Check sheet for the drawn part. Datum: minimum x, y, z corner. Units: mm. A direction names the side the tool comes from. Round coordinates to 2 decimals unless told otherwise and drop trailing zeros. Loops run counter-clockwise (first coordinate to the right, second up) from the corner with the lowest first, then second, coordinate; pieces in that order, holes last.
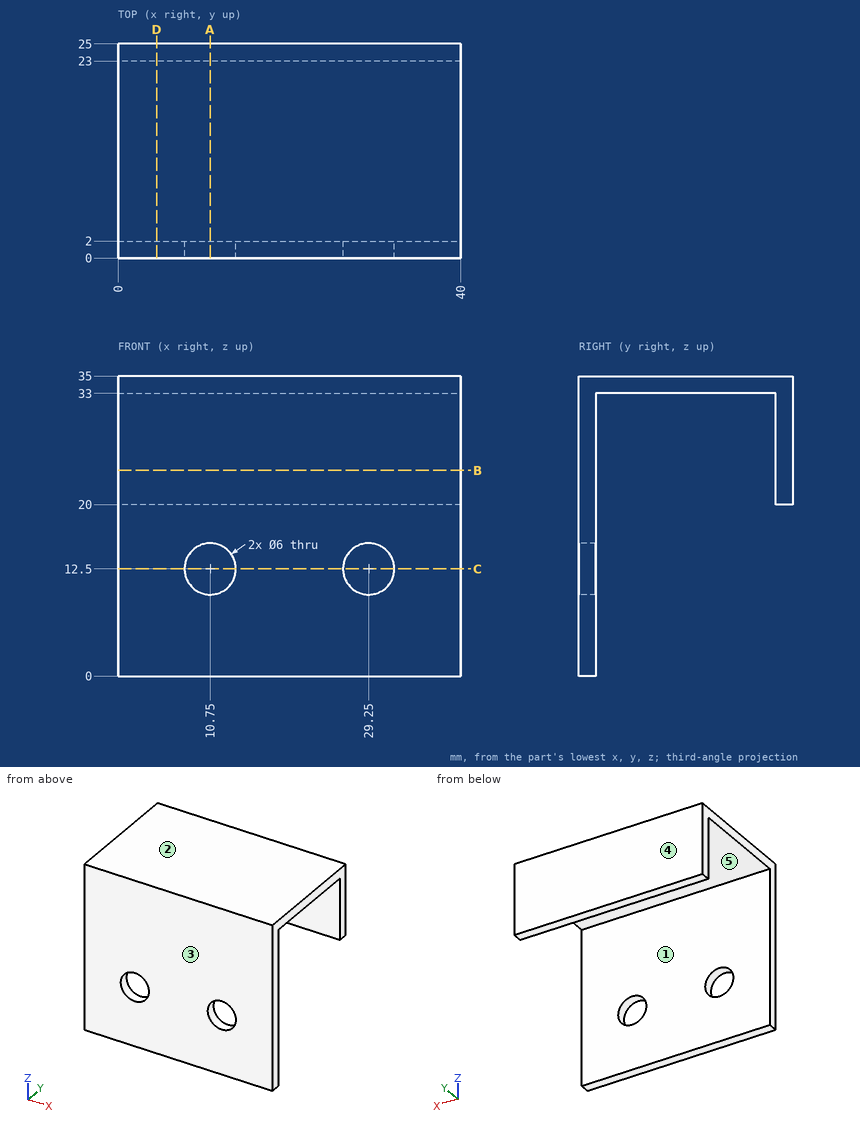
1) Gauge pin test, flat ends, axial feed: pin 1 (6 mm diameter, centred on x = 11.5, y = 11.5, fed in from -Z); pin 2 (1.5 mm diameter, centred on y = 22, z = 18.5, fed in from +X); pin 3 (0.6 mm diameter, centred on x = 20.5, y = 24, fed in from -Z). Record the tip position at first contact, or that the pin passes through.
Report:
pin 1: stops at z = 33
pin 2: passes through
pin 3: stops at z = 20
2) Sectioned sample at D-D, the plane x = 4.5. Record the cut outline in (y, z), then the cut area to 3 significant figures.
Report:
outline: (0, 0) - (2, 0) - (2, 33) - (23, 33) - (23, 20) - (25, 20) - (25, 35) - (0, 35) - close
area: 142 mm2
3) Access from +Z, -Z, +X, -X, +Y, -Y to the whole of each face (thin tool, end or side, straight path). Record for the marked faces 4 and 5.
Report:
face 4: +Z, -Z, +X, -X, +Y
face 5: -Z, +X, -X
4) Scan lines: line 1 along X through (y, z) = (0.5, 12.5); line 2 along Y through (x, z) = (6.5, 24); line 3 along Z through (x, y) = (29.25, 0.8). Record each from-to range of solid material in increasing order.
Report:
line 1: x = 0 to 7.75, 13.75 to 26.25, 32.25 to 40
line 2: y = 0 to 2, 23 to 25
line 3: z = 0 to 9.5, 15.5 to 35
5) Sectioned sample at A-A, the plane x = 10.75. Record the cut outline in (y, z).
Report:
outline: (0, 0) - (2, 0) - (2, 9.5) - (0, 9.5) - close; (0, 15.5) - (2, 15.5) - (2, 33) - (23, 33) - (23, 20) - (25, 20) - (25, 35) - (0, 35) - close
6) Sectioned sample at C-C, the plane z = 12.5. Record the cut outline in (x, y), then the cut area to 3 significant figures.
Report:
outline: (0, 0) - (7.75, 0) - (7.75, 2) - (0, 2) - close; (13.75, 0) - (26.25, 0) - (26.25, 2) - (13.75, 2) - close; (32.25, 0) - (40, 0) - (40, 2) - (32.25, 2) - close
area: 56.0 mm2
7) Mould release check, pull along Y, two halves, no side actions. Record for the marked faces 1, 2 and 3: +Y half, -Y half, draft (parallel to the pull), parting line (faces both ways), or undercut.
Report:
face 1: undercut
face 2: draft
face 3: -Y half
8) Sectioned sample at B-B, the plane z = 24. Record the cut outline in (x, y).
Report:
outline: (0, 0) - (40, 0) - (40, 2) - (0, 2) - close; (0, 23) - (40, 23) - (40, 25) - (0, 25) - close
